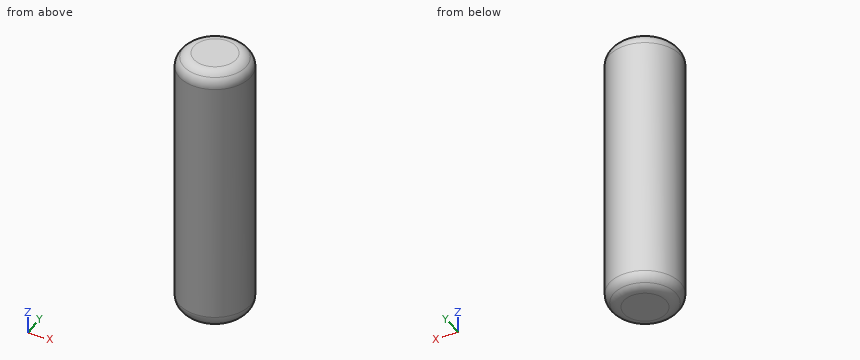
from build123d import *

# Parameters (mm, degrees)
SKETCH4_R           = 2
BOSS_EXTRUDE2_DEPTH = 15
SKETCH5_R           = 1.75
BOSS_EXTRUDE3_DEPTH = 0.25
FILLET3_R           = 0.75
SKETCH6_R           = 1.75
BOSS_EXTRUDE4_DEPTH = 0.25
FILLET4_R           = 0.75


with BuildPart() as part:
    # Sketch4 → Boss-Extrude2 (new body)
    with BuildSketch(Plane.XY):
        Circle(SKETCH4_R)
    extrude(amount=BOSS_EXTRUDE2_DEPTH)

    # Sketch5 → Boss-Extrude3 (add)
    with BuildSketch(Plane.XY.offset(15)):
        Circle(SKETCH5_R)
    extrude(amount=BOSS_EXTRUDE3_DEPTH)

    # Fillet3
    # the kernel refuses this fillet: 0.75 mm, written as the material it takes off along each edge
    with BuildSketch(Plane(origin=(0, 0, 15), x_dir=(1, 0, 0), z_dir=(0, -1, 0))) as fillet3_piece_1:
        with BuildLine():
            CenterArc((1.25, -0.559016994), FILLET3_R, 0, 48.189685104)
            Line((1.75, 0), (1.76, 0.01118034))
            ThreePointArc((1.76, 0.01118034), (1.875, 0.015), (2, 0.015))
            Line((2, 0.015), (2.015, 0))
            Line((2.015, 0), (2.015, -0.559016994))
            Line((2.015, -0.559016994), (2, -0.559016994))
        make_face()
    revolve(axis=Axis((0, 0, 15), (0, 0, 1)), mode=Mode.SUBTRACT)
    with BuildSketch(Plane(origin=(0, 0, 15.25), x_dir=(1, 0, 0), z_dir=(0, -1, 0))) as fillet3_piece_2:
        with BuildLine():
            CenterArc((1.190983006, -0.75), FILLET3_R, 41.810314896, 48.189685104)
            Line((1.190983006, 0), (1.190983006, 0.015))
            Line((1.190983006, 0.015), (1.75, 0.015))
            Line((1.75, 0.015), (1.765, 0))
            ThreePointArc((1.765, 0), (1.765, -0.125), (1.76118034, -0.24))
            Line((1.76118034, -0.24), (1.75, -0.25))
        make_face()
    revolve(axis=Axis((0, 0, 15.25), (0, 0, 1)), mode=Mode.SUBTRACT)

    # Sketch6 → Boss-Extrude4 (add)
    with BuildSketch(Plane(origin=(0, 0, 0), x_dir=(-1, 0, 0), z_dir=(0, 0, -1))):
        Circle(SKETCH6_R)
    extrude(amount=BOSS_EXTRUDE4_DEPTH)

    # Fillet4
    # the kernel refuses this fillet: 0.75 mm, written as the material it takes off along each edge
    with BuildSketch(Plane(origin=(0, 0, -0.25), x_dir=(-1, 0, 0), z_dir=(0, -1, 0))) as fillet4_piece_1:
        with BuildLine():
            CenterArc((1.190983006, -0.75), FILLET4_R, 41.810314896, 48.189685104)
            Line((1.190983006, 0), (1.190983006, 0.015))
            Line((1.190983006, 0.015), (1.75, 0.015))
            Line((1.75, 0.015), (1.765, 0))
            ThreePointArc((1.765, 0), (1.765, -0.125), (1.76118034, -0.24))
            Line((1.76118034, -0.24), (1.75, -0.25))
        make_face()
    revolve(axis=Axis((0, 0, -0.25), (0, 0, -1)), mode=Mode.SUBTRACT)
    with BuildSketch(Plane(origin=(0, 0, 0), x_dir=(1, 0, 0), z_dir=(0, -1, 0))) as fillet4_piece_2:
        with BuildLine():
            CenterArc((1.25, 0.559016994), FILLET4_R, 311.810314896, 48.189685104)
            Line((1.75, 0), (1.76, -0.01118034))
            ThreePointArc((1.76, -0.01118034), (1.875, -0.015), (2, -0.015))
            Line((2, -0.015), (2.015, 0))
            Line((2.015, 0), (2.015, 0.559016994))
            Line((2.015, 0.559016994), (2, 0.559016994))
        make_face()
    revolve(axis=Axis((0, 0, 0), (0, 0, 1)), mode=Mode.SUBTRACT)


solid = part.part
Check sheet for the modelled part. Datum: model origin and axes. Units: mm. Round coordinates to 2 decimals unless told otherwise and drop trailing zeros. Loops run counter-clockwise (first coordinate to the right, second up) from the corner with the lowest first, then second, coordinate; pieces in that order, holes last. Notation, with made-up numbers: M 88,-13.75 L 136,-13.75 A23 cw 136,0.25 Z; hole C 54.25,87 d9. An arc over 180 degrees is marked long. One line per question, with ' | ' between items. Start each with the question number.
Item 1: Scan lines: probe 1 along Z at (x, y) = (-1, -0.75); probe 2 along Z at (x, y) = (1.4, -1.05); probe 3 along Y at (x, z) = (1.15, 3.5). Record each from-to range of solid material in increasing order.
Item 2: Gauge pin test, flat ends, axial feed: pin 1 Ø1 at (y, z) = (1, 8.5) entering from +X; pin 2 Ø1.5 at (x, y) = (1, 1) entering from +Z; pin 3 Ø1.5 at (y, z) = (-1, 9.5) entering from -X. Record the tip position at first contact, or that the pin passes through.
Item 3: Section check A-A (z = 11.25). Record the boundary of the cut face in (x, y), and give its area (3 significant figures).
Worked out:
1) probe 1: -0.25 to 15.25 | probe 2: 0 to 15 | probe 3: -1.64 to 1.64
2) pin 1: x = 1.94 | pin 2: z = 15.25 | pin 3: x = -1.98
3) outline: C 0,0 d4 | area: 12.6 mm^2
